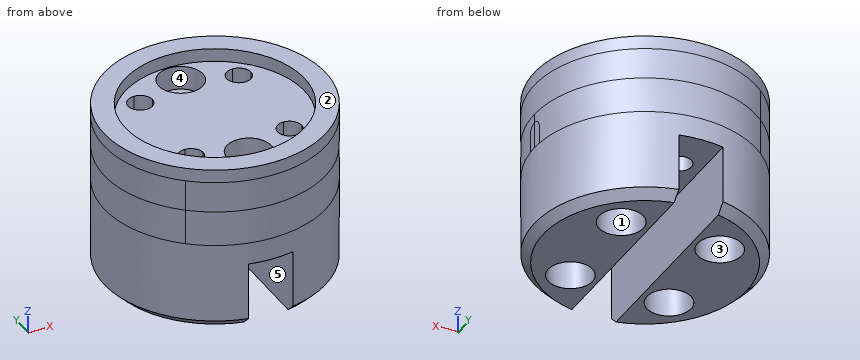
```python
from build123d import *
from build123d.topology import SkipClean

# Parameters (mm, degrees)
SKETCH1_R                                           = 25
BOSS_EXTRUDE1_DEPTH                                 = 15
CUT_EXTRUDE1_DEPTH                                  = 4
SKETCH3_R                                           = 2
CUT_EXTRUDE2_DEPTH                                  = 39.405728739
CUT_EXTRUDE3_DEPTH                                  = 4
FILLET1_R                                           = 0.5
SKETCH5_R                                           = 0.5
CUT_EXTRUDE4_DEPTH                                  = 8
F_5_5_5_5_DIAMETER_HOLE1_D                          = 5.5
CUT_EXTRUDE5_DEPTH                                  = 37.249138081
SKETCH9_R                                           = 25
SKETCH9_R_2                                         = 20.25
BOSS_EXTRUDE2_DEPTH                                 = 3
BOSS_EXTRUDE3_START                                 = 7
BOSS_EXTRUDE3_DEPTH                                 = 7
FILLET3_R                                           = 1
FILLET4_R                                           = 1
BOSS_EXTRUDE4_START                                 = -8
SKETCH11_R                                          = 25
SKETCH11_R_2                                        = 2.75
BOSS_EXTRUDE4_DEPTH                                 = 8
CBORE_FOR_M5_HEX_SOCKET_HEAD_CAP_SCR_2_COUNT        = 2
CBORE_FOR_M5_HEX_SOCKET_HEAD_CAP_SCR_2_PITCH        = 22.273863607
CBORE_FOR_M5_HEX_SOCKET_HEAD_CAP_SCR_3_COUNT        = 2
CBORE_FOR_M5_HEX_SOCKET_HEAD_CAP_SCR_3_PITCH        = 22.273863607
CBORE_FOR_M5_HEX_SOCKET_HEAD_CAP_SCR_4_COUNT        = 2
CBORE_FOR_M5_HEX_SOCKET_HEAD_CAP_SCR_4_PITCH        = 31.5
BOSS_EXTRUDE5_START                                 = 20
SKETCH15_R                                          = 25
SKETCH15_R_2                                        = 5
SKETCH15_R_3                                        = 5.025
BOSS_EXTRUDE5_DEPTH                                 = 20
CUT_EXTRUDE7_DEPTH                                  = 41.620192146
CUT_EXTRUDE7_DEPTH_BACK                             = 41.620192146
SKETCH16_W                                          = 10
SKETCH16_H                                          = 16.387019029
CBORE_FOR_M5_HEX_SOCKET_HEAD_CAP_SCREW2_D           = 5.5
CBORE_FOR_M5_HEX_SOCKET_HEAD_CAP_SCREW2_CBORE_D     = 10
CBORE_FOR_M5_HEX_SOCKET_HEAD_CAP_SCREW2_CBORE_DEPTH = 5.4
CHAMFER1_SIZE                                       = 2


with BuildPart() as part:
    # Sketch1 → Boss-Extrude1 (new body)
    with BuildSketch(Plane.XY):
        Circle(SKETCH1_R)
    extrude(amount=BOSS_EXTRUDE1_DEPTH)

    # Sketch2 → Cut-Extrude1 (cut)
    with BuildSketch(Plane(origin=(0, 0, 0), x_dir=(-1, 0, 0), z_dir=(0, 0, -1))):
        Polygon((0, 4), (2.3, 4), (2.3, 4.75), (13.4, 4.75), (13.4, 3), (16.4, 3), (16.4, 25), (28.321861399, 25), (28.321861399, -25), (16.4, -25), (16.4, -3), (13.4, -3), (13.4, -4.75), (2.3, -4.75), (2.3, -4), (0, -4), (0, -2), (-29.291687819, -2), (-29.291687819, 2), (0, 2), align=None)
    extrude(amount=-CUT_EXTRUDE1_DEPTH, mode=Mode.SUBTRACT)

    # Sketch3 → Cut-Extrude2 (cut, through all)
    with BuildSketch(Plane.ZY):
        with Locations((4, 0)):
            Circle(SKETCH3_R)
    extrude(amount=-CUT_EXTRUDE2_DEPTH, mode=Mode.SUBTRACT)

    # Sketch4 → Cut-Extrude3 (cut)
    with BuildSketch(Plane(origin=(0, 0, 4), x_dir=(-1, 0, 0), z_dir=(0, 0, -1))):
        with BuildLine():
            Line((0, -2), (0, -4))
            Line((0, -4), (2.3, -4))
            Line((2.3, -4), (2.3, -4.75))
            Line((2.3, -4.75), (13.4, -4.75))
            Line((13.4, -4.75), (13.4, -3))
            Line((13.4, -3), (16.4, -3))
            Line((16.4, -3), (16.4, -18.869022232))
            ThreePointArc((16.4, -18.869022232), (25, 0), (16.4, 18.869022232))
            Line((16.4, 18.869022232), (16.4, 3))
            Line((16.4, 3), (13.4, 3))
            Line((13.4, 3), (13.4, 4.75))
            Line((13.4, 4.75), (2.3, 4.75))
            Line((2.3, 4.75), (2.3, 4))
            Line((2.3, 4), (0, 4))
            Line((0, 4), (0, 2))
            Line((0, 2), (0, -2))
        make_face()
    extrude(amount=-CUT_EXTRUDE3_DEPTH, mode=Mode.SUBTRACT)

    # Fillet1
    fillet1_edges = [part.edges().sort_by_distance(p)[0] for p in [
        (0, -2, 2),
        (0, 2, 2),
        (0, 0, 6),
    ]]
    fillet(fillet1_edges, radius=FILLET1_R)

    # Sketch5 → Cut-Extrude4 (cut)
    with BuildSketch(Plane(origin=(0, 0, 0), x_dir=(-1, 0, 0), z_dir=(0, 0, -1))):
        with Locations((0, 4)):
            Circle(SKETCH5_R)
        with Locations((13.4, 4.75)):
            Circle(SKETCH5_R)
        with Locations((0, -4)):
            Circle(SKETCH5_R)
        with Locations((13.4, -4.75)):
            Circle(SKETCH5_R)
    extrude(amount=-CUT_EXTRUDE4_DEPTH, mode=Mode.SUBTRACT)

    # Ø5.5 (5.5) Diameter Hole1 (through all)
    with Locations(Plane(origin=(0, 0, 0), x_dir=(-1, 0, 0), z_dir=(0, 0, -1))):
        with Locations((-11.136931804, 11.136931804), (11.136931804, 11.136931804), (-11.136931804, -11.136931804), (11.136931804, -11.136931804)):
            Hole(F_5_5_5_5_DIAMETER_HOLE1_D / 2)

    # Sketch8 → Cut-Extrude5 (cut, through all)
    with BuildSketch(Plane(origin=(0, 0, 8), x_dir=(-1, 0, 0), z_dir=(0, 0, -1))):
        with BuildLine():
            Line((16.4, 18.869022232), (16.4, -18.869022232))
            ThreePointArc((16.4, -18.869022232), (25, 0), (16.4, 18.869022232))
        make_face()
    extrude(amount=-CUT_EXTRUDE5_DEPTH, mode=Mode.SUBTRACT)

    # Sketch9 → Boss-Extrude2 (add)
    with BuildSketch(Plane.XY.offset(15)):
        with Locations(Location((0, 0, 0), (0, 0, 130.99551881))):
            Circle(SKETCH9_R)
        with Locations(Location((0, 0, 0), (0, 0, 144.083871109))):
            Circle(SKETCH9_R_2, mode=Mode.SUBTRACT)
    extrude(amount=BOSS_EXTRUDE2_DEPTH)

    # Sketch10 → Boss-Extrude3 (add)
    with SkipClean():  # the faces are left unmerged after this step: merging them gives an invalid solid
        with BuildSketch(Plane(origin=(0, 0, 15), x_dir=(-1, 0, 0), z_dir=(0, 0, -1)).offset(BOSS_EXTRUDE3_START)):
            with BuildLine():
                Line((16.4, 18.869022232), (16.4, -18.869022232))
                ThreePointArc((16.4, -18.869022232), (25, 0), (16.4, 18.869022232))
            make_face()
        extrude(amount=-BOSS_EXTRUDE3_DEPTH)

    # Fillet3
    # the kernel refuses this fillet: 1 mm, written as the material it adds along each edge
    with BuildSketch(Plane(origin=(-2.3, 4.75, 10.420614591), x_dir=(0, -1, 0), z_dir=(0, 0, -1)), Plane(origin=(-2.3, -4.75, 0), x_dir=(0, 1, 0), z_dir=(0, 0, 1))) as fillet3_piece_1:
        with BuildLine():
            CenterArc((1, 0.968245837), FILLET3_R, 180, 75.522487814)
            Line((0, 0.968245837), (-0.02, 0.968245837))
            Line((-0.02, 0.968245837), (-0.02, 0))
            Line((-0.02, 0), (0, -0.02))
            ThreePointArc((0, -0.02), (0.375, -0.02), (0.745, -0.019364917))
            Line((0.745, -0.019364917), (0.75, 0))
        make_face()
    extrude(amount=10.420614591)

    # Fillet4
    # the kernel refuses this fillet: 1 mm, written as the material it takes off along each edge
    with BuildSketch(Plane(origin=(-2.3, 4, 8), x_dir=(-0.44744459774228634, 0.894311652586079, 0), z_dir=(0, 0, -1)), Plane(origin=(-2.3, -4, -1.482509158), x_dir=(-0.44744459774200684, -0.8943116525862188, 0), z_dir=(0, 0, 1))) as fillet4_piece_1:
        with BuildLine():
            CenterArc((0.628975367, 0.977774684), FILLET4_R, 206.57984982, 51.317812547)
            Line((-0.265336285, 0.530330086), (0, 0))
            ThreePointArc((0, 0), (0.209658456, 0.022225316), (0.419316911, 0))
        make_face()
    extrude(amount=9.482509158, mode=Mode.SUBTRACT)

    # Sketch11 → Boss-Extrude4 (add)
    with BuildSketch(Plane(origin=(0, 0, 0), x_dir=(-1, 0, 0), z_dir=(0, 0, -1)).offset(BOSS_EXTRUDE4_START)):
        with Locations(Location((0, 0, 0), (0, 0, 180))):
            Circle(SKETCH11_R)
        with Locations((11.136931804, -11.136931804)):
            Circle(SKETCH11_R_2, mode=Mode.SUBTRACT)
        with Locations((11.136931804, 11.136931804)):
            Circle(SKETCH11_R_2, mode=Mode.SUBTRACT)
        with Locations((-11.136931804, -11.136931804)):
            Circle(SKETCH11_R_2, mode=Mode.SUBTRACT)
        with Locations((-11.136931804, 11.136931804)):
            Circle(SKETCH11_R_2, mode=Mode.SUBTRACT)
    extrude(amount=BOSS_EXTRUDE4_DEPTH)

    # Sketch14 → CBORE for M5 Hex Socket Head Cap Screw1 (revolve, cut)
    with BuildSketch(Plane(origin=(11.136931804, -11.136931804, 0), x_dir=(0, 1, 0), z_dir=(1, 0, 0))):
        Polygon((0, 0), (0, 18), (2.75, 18), (2.75, 5.4), (5, 5.4), (5, 0.025), (5.025, 0), align=None)
    cbore_for_m5_hex_socket_head_cap_screw1 = revolve(axis=Axis((11.136931804, -11.136931804, -6.35), (0, 0, 1)), mode=Mode.SUBTRACT)

    # CBORE for M5 Hex Socket Head Cap Scr 2: CBORE for M5 Hex Socket Head Cap Screw1 ×2
    with Locations(*[(0, i * CBORE_FOR_M5_HEX_SOCKET_HEAD_CAP_SCR_2_PITCH, 0) for i in range(1, CBORE_FOR_M5_HEX_SOCKET_HEAD_CAP_SCR_2_COUNT)]):
        add(cbore_for_m5_hex_socket_head_cap_screw1, mode=Mode.SUBTRACT)

    # CBORE for M5 Hex Socket Head Cap Scr 3: CBORE for M5 Hex Socket Head Cap Screw1 ×2
    with Locations(*[(-i * CBORE_FOR_M5_HEX_SOCKET_HEAD_CAP_SCR_3_PITCH, 0, 0) for i in range(1, CBORE_FOR_M5_HEX_SOCKET_HEAD_CAP_SCR_3_COUNT)]):
        add(cbore_for_m5_hex_socket_head_cap_screw1, mode=Mode.SUBTRACT)

    # CBORE for M5 Hex Socket Head Cap Scr 4: CBORE for M5 Hex Socket Head Cap Screw1 ×2
    with Locations(*[Vector(-0.7071067811865435, 0.7071067811865516, 0) * (i * CBORE_FOR_M5_HEX_SOCKET_HEAD_CAP_SCR_4_PITCH) for i in range(1, CBORE_FOR_M5_HEX_SOCKET_HEAD_CAP_SCR_4_COUNT)]):
        add(cbore_for_m5_hex_socket_head_cap_screw1, mode=Mode.SUBTRACT)

    # Sketch15 → Boss-Extrude5 (add)
    with SkipClean():  # the faces are left unmerged after this step: merging them gives an invalid solid
        with BuildSketch(Plane(origin=(0, 0, 0), x_dir=(-1, 0, 0), z_dir=(0, 0, -1)).offset(BOSS_EXTRUDE5_START)):
            Circle(SKETCH15_R)
            with Locations((-11.136931804, -11.136931804)):
                Circle(SKETCH15_R_2, mode=Mode.SUBTRACT)
            with Locations((-11.136931804, 11.136931804)):
                Circle(SKETCH15_R_3, mode=Mode.SUBTRACT)
            with Locations((11.136931804, -11.136931804)):
                Circle(SKETCH15_R_2, mode=Mode.SUBTRACT)
            with Locations((11.136931804, 11.136931804)):
                Circle(SKETCH15_R_2, mode=Mode.SUBTRACT)
        extrude(amount=-BOSS_EXTRUDE5_DEPTH)
    add(part.part.scale(1), mode=Mode.REPLACE)  # the faces are merged on a copy

    # Sketch16 → Cut-Extrude7 (cut, two sides: drawn at the far end of the back side and taken through both)
    with BuildSketch(Plane(origin=(0, 0, 0), x_dir=(1, 0, 0), z_dir=(0, 1, 0)).offset(-CUT_EXTRUDE7_DEPTH_BACK)):
        with Locations((0, 13.193509515)):
            Rectangle(SKETCH16_W, SKETCH16_H)
    extrude(amount=CUT_EXTRUDE7_DEPTH + CUT_EXTRUDE7_DEPTH_BACK, mode=Mode.SUBTRACT)

    # CBORE for M5 Hex Socket Head Cap Screw2 (through all)
    with Locations(Plane.XY.offset(15)):
        with Locations((0, -15), (0, 15)):
            CounterBoreHole(CBORE_FOR_M5_HEX_SOCKET_HEAD_CAP_SCREW2_D / 2, CBORE_FOR_M5_HEX_SOCKET_HEAD_CAP_SCREW2_CBORE_D / 2, CBORE_FOR_M5_HEX_SOCKET_HEAD_CAP_SCREW2_CBORE_DEPTH)

    # Chamfer1
    chamfer1_edges = [part.edges().sort_by_distance(p)[0] for p in [
        (25, 0, -20),
        (-19.364916731, 15.811388301, -20),
    ]]
    chamfer(chamfer1_edges, length=CHAMFER1_SIZE)


solid = part.part
```
Verification items for the finished model (mm, model axes). Face numbers are marked on the shaded views. A direction names the side the tool comes from. Coordinates: 2 decimals unless noted, no trailing zeros. Loops run counter-clockwise (first coordinate to the right, second up) from the corner with the lowest first, then second, coordinate; pieces in that order, holes last. Notation, with made-up numbers: (78.5, 82) - (136.5, 82) arc R18 ccw to (136.5, 91) - close; hole circle Ø7 at (75.25, 33). An arc over 180 degrees is marked (long way). Answer as a JSON object with one key per item and string values.
(1) Access from +Z, -Z, +X, -X, +Y, -Y to the whole of each face (thin tool, end or side, straight path). Record for the marked faces 3, 4 and 5.
Response:
{"face 3": "-Z", "face 4": "+Z", "face 5": "-Z, +Y, -Y"}
(2) Cross-section at B-B, the plane z = 1.5. Record the boundary of the cut face in (x, y), then the cut area to 3 significant figures.
Response:
{"outline": "circle Ø50 at (0, 0); hole circle Ø10 at (-11.14, -11.14); hole circle Ø10 at (-11.14, 11.14); hole circle Ø5.5 at (0, -15); hole circle Ø5.5 at (0, 15); hole circle Ø10 at (11.14, -11.14); hole circle Ø10 at (11.14, 11.14)", "area": "1,600 mm²"}
(3) Cross-section at A-A, the plane z = -15. Record the boundary of the cut face in (x, y) (3 decimals), then the cut area to 3 significant figures.
Response:
{"outline": "(-5, -24.495) - (-5, 24.495) arc R25 ccw to start; (5, -24.495) arc R25 ccw to (5, 24.495) - close; hole circle Ø10 at (-11.137, -11.137); hole circle Ø10 at (-11.137, 11.137); hole circle Ø10.05 at (11.137, 11.137); hole circle Ø10 at (11.137, -11.137)", "area": "1,150 mm²"}
(4) Go/stop test with flat-tipped pins: pin 1 Ø12 at (y, z) = (-13, -3.5) entering from +X; pin 2 Ø4.5 at (y, z) = (3, -15.5) entering from +X; pin 3 Ø3.5 at (x, y) = (0, -15) entering from -Z; pin 4 Ø2 at (x, z) = (-8, -1) entering from -Y. Record where each tip stops, or that it passes through.
Response:
{"pin 1": "stops at x = 24", "pin 2": "stops at x = 24.99", "pin 3": "passes through", "pin 4": "stops at y = -24"}
(5) Scan lines: line 1 along Y through (x, z) = (-12.5, 0); line 2 along X through (y, z) = (-11, -11.5); line 3 along X through (y, z) = (-10.5, 12.5). Record each from-to range of solid material in increasing order.
Response:
{"line 1": "y = -21.65 to -15.97, -6.3 to 6.3, 15.97 to 21.65", "line 2": "x = -22.45 to -16.14, -6.14 to -5, 5 to 6.14, 16.14 to 22.45", "line 3": "x = -22.69 to -13.81, -8.46 to -2.18, 2.18 to 8.46, 13.81 to 22.69"}
(6) Cross-section at D-D, the plane z = 11.5. Record the boundary of the cut face in (x, y), then the cut area to 3 significant figures.
Response:
{"outline": "circle Ø50 at (0, 0); hole circle Ø5.5 at (-11.14, -11.14); hole circle Ø5.5 at (-11.14, 11.14); hole circle Ø10 at (0, -15); hole circle Ø10 at (0, 15); hole circle Ø5.5 at (11.14, -11.14); hole circle Ø5.5 at (11.14, 11.14)", "area": "1,710 mm²"}
(7) Cross-section at C-C, the plane x = 0. Record the boundary of the cut face in (y, z), then the cut area to 3 significant figures.
Response:
{"outline": "(-25, -5) - (-17.75, -5) - (-17.75, 9.6) - (-20, 9.6) - (-20, 15) - (-20.25, 15) - (-20.25, 18) - (-25, 18) - close; (-12.25, -5) - (12.25, -5) - (12.25, 9.6) - (10, 9.6) - (10, 15) - (-10, 15) - (-10, 9.6) - (-12.25, 9.6) - close; (17.75, -5) - (25, -5) - (25, 18) - (20.25, 18) - (20.25, 15) - (20, 15) - (20, 9.6) - (17.75, 9.6) - close", "area": "760 mm²"}
(8) Mould release check, pull along X, two halves, no side actions. Record for the marked faces 1 and 2: pulls with the +X half, pulls with the -X half, needs draft (parallel to the pull), parting line crosses it, or undercut.
Response:
{"face 1": "undercut", "face 2": "needs draft"}
